```python
from build123d import *

# Parameters (mm, degrees)
F0_W     = 30
F0_H     = 10
F1_DEPTH = 30
F3_D     = 5
F3_DEPTH = 25
F3_TIP   = 1.5021515476
F4_R     = 5
F5_R     = 10
F6_DEPTH = 1.5


with BuildPart() as f1:
    # F0 (on Top) → F1 (new body)
    with BuildSketch(Plane.XY):
        Rectangle(F0_W, F0_H)
        Polygon((-15, 5), (15, 5), (58.3012701892, 80), (28.3012701892, 80), align=None)
        with Locations((43.3012701892, 85)):
            Rectangle(F0_W, F0_H)
    extrude(amount=F1_DEPTH)

    # F3
    with Locations(Plane.XZ.offset(5)):
        with Locations((0, 22.5), (0, 7.5)):
            Hole(F3_D / 2, depth=F3_DEPTH)
            with Locations((0, 0, -(F3_DEPTH + F3_TIP / 2))):  # 118° drill point
                Cone(0, F3_D / 2, F3_TIP, mode=Mode.SUBTRACT)

    # F4
    f4_edges = [f1.edges().sort_by_distance(p)[0] for p in [
        (15, 0, 0),
        (36.650635, 42.5, 0),
        (15, 0, 30),
        (36.650635, 42.5, 30),
        (-15, 0, 30),
        (6.650635, 42.5, 30),
        (28.30127, 85, 30),
        (58.30127, 85, 30),
        (58.30127, 85, 0),
        (28.30127, 85, 0),
        (6.650635, 42.5, 0),
        (-15, 0, 0),
        (58.30127, 80, 15),
        (15, 5, 15),
        (-15, 5, 15),
        (28.30127, 80, 15),
    ]]
    fillet(f4_edges, radius=F4_R)

    # F5 (on face) → F6 (cut)
    with BuildSketch(Plane(origin=(0, 90, 0), x_dir=(-1, 0, 0), z_dir=(0, 1, 0))):
        with Locations((-43.3012701892, 15)):
            Circle(F5_R)
    extrude(amount=-F6_DEPTH, mode=Mode.SUBTRACT)


solid = f1.part
```
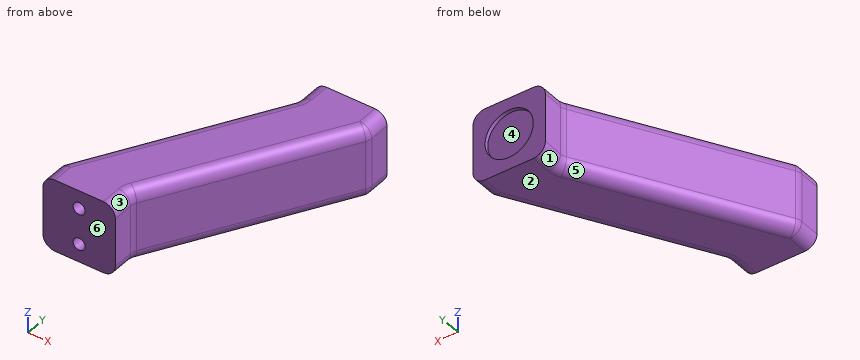
Work out the finished part from the listing and answer in its coordinate system (mm). Face numbers are marked on the shaded views. A direction names the side the tool comes from. Round coordinates to 2 decimals unless told otherwise and drop trailing zeros. Write each loop counter-clockwise with the first axis right and the second up, starting at its lowest first coordinate (ties: lowest second). Pieces come first, ordered by that corner, then holes.
1) Flat-ended cylindrical pins translate along their axes: P1, Ø8, axis at y = 73.5, z = 10, coming from the -X side; P2, Ø1.5, axis at x = -0.5, z = 10.5, coming from the +Y side; P3, Ø5, axis at y = 46.5, z = 5.5, coming from the +X side. Find the tip coordinate at first contact, or state that the pin passes through.
2) Consider probe 1 along Z at (x, y) = (0, 14.75); probe 2 along X at (y, z) = (11.5, 7.5); probe 3 along X at (y, z) = (11.75, 22.5). Determine where each line is inside the solid, lowest interval first.
3) Which of the six approach directions +Z, -Z, +X, -X, +Y, -Y give full straight-line access (tool end or side, diameter ignored) to the marked faces 1 and 2?
4) Determine the mould class of the marked faces 3, 4, 5 and 6 for opening direction Z: pulls with the +Z half, pulls with the -Z half, needs draft (parallel to the pull), parting line crosses it, or undercut.
5) A cutting plane is placed at B-B on z = 3.25. Determine the outline of the cut face in (x, y).
6) A cutting plane is placed at A-A on z = 15. Determine the outline of the cut face in (x, y).
Entries:
1. P1: stops at x = 22.24
1. P2: stops at y = 31.41
1. P3: stops at x = 40.4
2. probe 1: z = 0 to 5, 10 to 20, 25 to 30
2. probe 2: x = -11.25 to -2.5, 2.5 to 18.75
2. probe 3: x = -11.1 to -2.5, 2.5 to 18.9
3. face 1: -Z, -X, +Y
3. face 2: -Z, +X, -X, +Y, -Y
4. face 3: pulls with the +Z half
4. face 4: undercut
4. face 5: pulls with the -Z half
4. face 6: needs draft
5. outline: (-14.68, -5) - (14.68, -5) - (14.68, 3.66) arc R5.32 cw to (15.4, 6.32) - (57.36, 79) arc R4.68 ccw to (57.99, 81.34) - (57.99, 90) - (28.62, 90) - (28.62, 81.34) arc R5.32 cw to (27.91, 78.68) - (-14.06, 6) arc R4.68 ccw to (-14.68, 3.66) - close
6. outline: (-15, -5) - (15, -5) - (15, 3.66) arc R5 cw to (15.67, 6.16) - (57.63, 78.84) arc R5 ccw to (58.3, 81.34) - (58.3, 90) - (53.3, 90) - (53.3, 88.5) - (33.3, 88.5) - (33.3, 90) - (28.3, 90) - (28.3, 81.34) arc R5 cw to (27.63, 78.84) - (-14.33, 6.16) arc R5 ccw to (-15, 3.66) - close
